Build history of the part. All positions in model axes, mm. A direction names the side the tool comes from. Give positions to 0.01 mm unless a question says otherwise; leave off trailing zeros. Order: outer loops, then holes, each group sorted by start corner. A loop starts at its lowest first (then second) coordinate and runs counter-clockwise, first axis right, second up. Notation, with made-up numbers: M 52.25,33 L 79.25,33 A15 cw 79.25,58 Z; hole C 84,-35 d6. An arc over 180 degrees is marked long. Answer as CSV lines item,"result".
from build123d import *

# Parameters (mm, degrees)
F2_R     = 25.4
F3_DEPTH = 127
F4_W     = 29.586202
F4_H     = 18.928807
F5_DEPTH = 127
F6_SIZE2 = 5.08
F6_SIZE  = 5.08


with BuildPart() as f1:
    # F0 (on Front) → F1 (revolve)
    with BuildSketch(Plane.XZ):
        Polygon((55.335713, 50.8), (-46.264287, 50.8), (-46.264287, 0), (12.566184, 0), (55.335713, 0), align=None)
    revolve(axis=Axis((4.535713, 0, 0), (1, 0, 0)))

    # F2 (on Right) → F3 (join)
    with BuildSketch(Plane.YZ):
        Circle(F2_R)
    extrude(amount=F3_DEPTH)

    # F4 (on Front) → F5 (join)
    with BuildSketch(Plane.XZ):
        with Locations((-12.207311, -9.464403)):
            Rectangle(F4_W, F4_H)
    extrude(amount=F5_DEPTH)

    # F6
    f6_edges = [f1.edges().sort_by_distance(p)[0] for p in [
        (2.58579, -127, -9.464404),
        (-12.207311, -127, 0),
        (-27.000412, -127, -9.464404),
        (-12.207311, -127, -18.928807),
    ]]
    chamfer(f6_edges, length=F6_SIZE, length2=F6_SIZE2)


solid = f1.part
Item 1: Band-saw the part on D-D (y = -86). Give the cut face in (x, z).
Geometry says:
outline,"M -27,-18.93 L 2.59,-18.93 L 2.59,0 L -27,0 Z"
Item 2: Band-saw the part on A-A (y = 0). Give the cut face in (x, z), and give its area (3 significant figures).
Geometry says:
outline,"M -46.26,-50.8 L 55.34,-50.8 L 55.34,-25.4 L 127,-25.4 L 127,25.4 L 55.34,25.4 L 55.34,50.8 L -46.26,50.8 Z"
area,"14,000 mm2"
Item 3: Band-saw the part on B-B (z = 16.5). Give the cut face in (x, y), and give its area (3 significant figures).
Geometry says:
outline,"M -46.26,-48.05 L 55.34,-48.05 L 55.34,-19.31 L 127,-19.31 L 127,19.31 L 55.34,19.31 L 55.34,48.05 L -46.26,48.05 Z"
area,"12,500 mm2"
Item 4: Drop flat-ended pins along their axis: pin 1 (12 mm diameter, centred on x = 45.5, z = -2.5, fed in from -Y); pin 2 (15 mm diameter, centred on y = -91.5, z = -7, fed in from -X); pin 3 (6 mm diameter, centred on x = -23, z = 23.5, fed in from +Y). Give the stop position or say it passes through.
Geometry says:
pin 1,"stops at y = -50.8"
pin 2,"stops at x = -27"
pin 3,"stops at y = 46.48"
Item 5: Probe line 1 along X through (y, z) = (22.5, 45.5); line 2 along Z through (x, y) = (-26, -76); line 3 along Z through (x, y) = (-28, 16). List the from-to ranges inside material, lowest first. Write a range as from..to.
Geometry says:
line 1,"x = -46.26..55.34"
line 2,"z = -18.93..0"
line 3,"z = -48.21..48.21"
Item 6: Band-saw the part on C-C (x = 77.5). Give the cut face in (y, z), and give its area (3 significant figures).
Geometry says:
outline,"C 0,0 d50.8"
area,"2,030 mm2"
Item 7: 3-axis set-ups, long thin cutter, end or side, ignore diameter. For faces 1 (the flat face through (-12, -84, -18.929)), 2 (the flat face through (-12, -86, 0)), 3 (the cylindrical face through (90.666, -5.506, -24.796)): which of +Z, -Z, +X, -X, +Y, -Y reach the whole face in a straight line?
Geometry says:
face 1,"-Z, +X, -X, -Y"
face 2,"+Z, +X, -X, -Y"
face 3,"+X"
